from build123d import *

# Parameters (mm, degrees)
BOSS_EXTRUDE1_DEPTH = 21.6
CUT_EXTRUDE1_REACH  = 23.6
SKETCH2_R           = 12
SKETCH3_OUTSIDE_W   = 135.272
SKETCH3_OUTSIDE_H   = 141.702
SKETCH3_OUTSIDE_R   = 20.784609691
CUT_EXTRUDE2_DEPTH  = 22.6
CUT_EXTRUDE2_TAPER  = 60


with BuildPart() as part:
    # Sketch1 → Boss-Extrude1 (new body)
    with BuildSketch(Plane(origin=(0, 0, 0), x_dir=(0, 0, -1), z_dir=(1, 0, 0))):
        Polygon((0, 24), (-20.784609691, 12), (-20.784609691, -12), (0, -24), (20.784609691, -12), (20.784609691, 12), align=None)
    extrude(amount=-BOSS_EXTRUDE1_DEPTH)

    # Sketch2 → Cut-Extrude1 (cut, up to next)
    with BuildSketch(Plane(origin=(0, 0, 0), x_dir=(0, 0, -1), z_dir=(1, 0, 0)), mode=Mode.PRIVATE) as cut_extrude1_sk1:
        Circle(SKETCH2_R)
    cut_extrude1_tool1 = extrude(cut_extrude1_sk1.sketch, amount=-CUT_EXTRUDE1_REACH, mode=Mode.PRIVATE) & part.part
    add(cut_extrude1_tool1.solids().sort_by_distance((0, 0, 0))[0], mode=Mode.SUBTRACT)

    # Sketch3 outside → Cut-Extrude2 (cut, through all)
    with BuildSketch(Plane(origin=(0, 0, 0), x_dir=(0, 0, -1), z_dir=(1, 0, 0))):
        Rectangle(SKETCH3_OUTSIDE_W, SKETCH3_OUTSIDE_H)
        Circle(SKETCH3_OUTSIDE_R, mode=Mode.SUBTRACT)
    extrude(amount=-CUT_EXTRUDE2_DEPTH, taper=CUT_EXTRUDE2_TAPER, mode=Mode.SUBTRACT)


solid = part.part
Geometry check sheet. Reference: the model listing, model coordinates, mm. Round coordinates to 2 decimals unless told otherwise and drop trailing zeros. Loops run counter-clockwise (first coordinate to the right, second up) from the corner with the lowest first, then second, coordinate; pieces in that order, holes last.
Item 1: Thickness scan on line 1 (Y direction, x = -6.5, z = 0); line 2 (Y direction, x = -8.5, z = 3.5); line 3 (Z direction, x = -3.25, y = -9). Record the ranges inside material, lowest first.
Item 2: Gauge pin test, flat ends, axial feed: pin 1 (6 mm diameter, centred on x = -15, z = 5, fed in from +Y); pin 2 (3 mm diameter, centred on x = -6, y = 16.5, fed in from +Z); pin 3 (3 mm diameter, centred on x = -17.5, z = -10, fed in from -Y). Record the tip position at first contact, or that the pin passes through.
Item 3: Cross-section at A-A on x = -19.25. Record the boundary of the cut face in (y, z).
Item 4: Mould release check, pull along Z, two halves, no side actions. Record for faces 1 (the flat face through (-10.649, -17.916, 10.538)), 2 (the cylindrical face through (-10.65, 0.53, 11.99)), 3 (the conical face through (-0.451, 21.566, 0.053)), 4 (the conical face through (-0.45, -10.74, -18.7)): pulls with the +Z half, pulls with the -Z half, needs draft (parallel to the pull), parting line crosses it, or undercut.
Answer sheet:
1. line 1: y = -24 to -12, 12 to 24
1. line 2: y = -21.98 to -11.48, 11.48 to 21.98
1. line 3: z = -20.78 to -7.94, 7.94 to 20.78
2. pin 1: stops at y = 22.85
2. pin 2: stops at z = 15.59
2. pin 3: stops at y = -19.09
3. outline: (-24, 0) - (-12, -20.78) - (12, -20.78) - (24, 0) - (12, 20.78) - (-12, 20.78) - close; hole circle Ø24 at (0, 0)
4. face 1: pulls with the +Z half
4. face 2: undercut
4. face 3: parting line crosses it
4. face 4: pulls with the -Z half
